Build history of the part. All positions in model axes, mm. Round coordinates to 2 decimals unless told otherwise and drop trailing zeros. Write each loop counter-clockwise with the first axis right and the second up, starting at its lowest first coordinate (ties: lowest second). Pieces come first, ordered by that corner, then holes.
Autodesk Inventor part; units mm, degrees
ref_plane "YZ Plane" through (0, 0, 0) normal (1, 0, 0) x (0, 1, 0)
ref_plane "XZ Plane" through (0, 0, 0) normal (0, 1, 0) x (-1, 0, 0)
ref_plane "XY Plane" through (0, 0, 0) normal (0, 0, 1) x (1, 0, 0)
sketch "Sketch_1" plane through (0, 0, 0) normal (0, 0, 1) x (1, 0, 0)
  line L0 (-50, 25) -> (-50, 0)
  line L1 (-50, 0) -> (50, 0)
  line L2 (50, 0) -> (50, 25)
  line L3 (50, 25) -> (25, 75)
  line L4 (25, 75) -> (-25, 75)
  line L5 (-25, 75) -> (-50, 25)
  circle A0 centre (37.5, 12.5) radius 3.175
  circle A1 centre (12.5, 12.5) radius 3.175
  circle A2 centre (12.5, 37.5) radius 3.175
  circle A3 centre (12.5, 62.5) radius 3.175
  circle A4 centre (-12.5, 37.5) radius 3.175
  circle A5 centre (-12.5, 12.5) radius 3.175
  circle A6 centre (-12.5, 62.5) radius 3.175
  circle A7 centre (-37.5, 12.5) radius 3.175
extrude "Extrusion1" add sketch "Sketch_1" along normal blind 4
properties part number "25-4155"
1) Slice it at B-B (x = 37.5). Write the cut outline in (y, z) (3 decimals), plus the area to 3 significant figures.
Results:
outline: (0, 0) - (9.325, 0) - (9.325, 4) - (0, 4) - close; (15.675, 0) - (50, 0) - (50, 4) - (15.675, 4) - close
area: 175 mm2
2) Slice it at A-A (y = 62.5). Write the cut outline in (x, z) (3 decimals), plus the area to 3 significant figures.
Results:
outline: (-31.25, 0) - (-15.675, 0) - (-15.675, 4) - (-31.25, 4) - close; (-9.325, 0) - (9.325, 0) - (9.325, 4) - (-9.325, 4) - close; (15.675, 0) - (31.25, 0) - (31.25, 4) - (15.675, 4) - close
area: 199 mm2
3) Slice it at C-C (y = 12.5). Write the cut outline in (x, z) (3 decimals).
Results:
outline: (-50, 0) - (-40.675, 0) - (-40.675, 4) - (-50, 4) - close; (-34.325, 0) - (-15.675, 0) - (-15.675, 4) - (-34.325, 4) - close; (-9.325, 0) - (9.325, 0) - (9.325, 4) - (-9.325, 4) - close; (15.675, 0) - (34.325, 0) - (34.325, 4) - (15.675, 4) - close; (40.675, 0) - (50, 0) - (50, 4) - (40.675, 4) - close
4) Slice it at D-D (z = 3.25). Count the separate pieces of the cut face and the enclosed holes in it, plus the area to 3 significant figures.
Results:
separate pieces: 1
enclosed holes: 8
area: 6,000 mm2
5) Mould opens along X. For faces 1 (the flat face through (-50, 13, 2)), 2 (the flat face through (37.7, 49.6, 2)), 3 (the cylindrical face through (-11, 15.3, 2)) say: released by +X, released by -X, zero draft, split by the parting line, or undercut.
Results:
face 1: released by -X
face 2: released by +X
face 3: undercut
6) Wall check: L1, parallel to Y at x = 12.5, z = 1.8 (3 decimals); L2, parallel to Y at x = 10, z = 2.35; L3, parallel to Y at x = 37.5, z = 2.9 (3 decimals). Give the ranges that are in metal, low to high.
Results:
L1: y = 0 to 9.325, 15.675 to 34.325, 40.675 to 59.325, 65.675 to 75
L2: y = 0 to 10.54, 14.46 to 35.54, 39.46 to 60.54, 64.46 to 75
L3: y = 0 to 9.325, 15.675 to 50
